Check sheet for the modelled part. Datum: model origin and axes. Units: mm. Give positions to 0.01 mm unless a question says otherwise; leave off trailing zeros. Write each loop counter-clockwise with the first axis right and the second up, starting at its lowest first coordinate (ties: lowest second). Pieces come first, ordered by that corner, then holes. Notation, with made-up numbers: (10.5, 29) -> (18.5, 29) arc R31 cw to (18.5, 56) -> close; hole circle Ø2 at (22, 77). An arc over 180 degrees is marked (long way). Write each question's results on one line, items separated by ' | '. Start each with the question number.
```python
from build123d import *

# Parameters (mm, degrees)
TD_SKETCH_R                             = 0.79248
TL_FEATURE_DEPTH                        = 21.0312
TDF_STD_SKETCH_W                        = 2.09296
TDF_STD_SKETCH_H                        = 2.09296
TDF_STD_FEATURE_DEPTH                   = 22.061040395
ISA_20_STD_FEATURE_DEPTH                = 22.061040395
ISA_20_STD_FEATURE_DEPTH_BACK           = 22.061040395
VW_STD_FEATURE_DEPTH                    = 22.061040395
VW_STD_FEATURE_DEPTH_BACK               = 22.061040395
F_10BA_STD_FEATURE_DEPTH                = 22.061040503
F_10BA_STD_FEATURE_DEPTH_BACK           = 22.061040503
FRO_STD_FEATURE_DEPTH                   = 22.061040395
FRO_STD_FEATURE_DEPTH_BACK              = 22.061040395
C_STD_FEATURE_DEPTH                     = 22.061040395
C_STD_FEATURE_DEPTH_BACK                = 22.061040395
ERW_STD_FEATURE_DEPTH                   = 0.01905
H_STD_FEATURE_REACH                     = 22.896
H_STD_SKETCH_R                          = 0.01905
H_STD_SKETCH_3_R                        = 0.01905
FUNNEL_FINAL_DIAMETRE_STD_FEATURE_DEPTH = 2.499995
FUNNEL_FINAL_DIAMETRE_STD_FEATURE_DRAFT = -22.5
ROUND_BR_STD_FEATURE_START              = -1
ROUND_BR_STD_FEATURE_DEPTH              = 1.009339363


with BuildPart() as part:
    # TD_sketch → TL_feature (new body)
    with BuildSketch(Plane(origin=(0, 0, 0), x_dir=(1, 0, 0), z_dir=(0, 1, 0))):
        with Locations(Location((0, 0, 0), (0, 0, 270))):
            Circle(TD_SKETCH_R)
    extrude(amount=TL_FEATURE_DEPTH)

    # TDF_STD_sketch → TDF_STD_feature (cut, through all)
    with BuildSketch(Plane(origin=(0, 0, 0), x_dir=(1, 0, 0), z_dir=(0, 1, 0))):
        with Locations((-1.4224, 0)):
            Rectangle(TDF_STD_SKETCH_W, TDF_STD_SKETCH_H)
    extrude(amount=TDF_STD_FEATURE_DEPTH, mode=Mode.SUBTRACT)

    # ISA_20_STD_sketch → ISA_20_STD_feature (cut, two sides: drawn at the far end of the back side and taken through both)
    with BuildSketch(Plane(origin=(0, 0, 0), x_dir=(0, 0, -1), z_dir=(1, 0, 0)).offset(-ISA_20_STD_FEATURE_DEPTH_BACK)):
        Polygon((-12.946999885, 73.253224398), (-3.738847997, 21.0312), (-0.03048, 0), (0.03048, 0), (3.738847997, 21.0312), (12.946999885, 73.253224398), (12.946999885, -32.802042202), (-12.946999885, -32.802042202), align=None)
    extrude(amount=ISA_20_STD_FEATURE_DEPTH + ISA_20_STD_FEATURE_DEPTH_BACK, mode=Mode.SUBTRACT)

    # VW_STD_sketch → VW_STD_feature (cut, two sides: drawn at the far end of the back side and taken through both)
    with BuildSketch(Plane(origin=(0, 0, 0), x_dir=(0, 0, -1), z_dir=(1, 0, 0)).offset(-VW_STD_FEATURE_DEPTH_BACK)):
        with BuildLine():
            Line((-70.448918022, 70.704723144), (-20.775394878, 21.0312))
            Line((-20.775394878, 21.0312), (-0.087997439, 0.343802561))
            ThreePointArc((-0.087997439, 0.343802561), (-0.060467299, 0.302600796), (-0.0508, 0.254))
            Line((-0.0508, 0.254), (-0.0508, 0))
            Line((-0.0508, 0), (0.0508, 0))
            Line((0.0508, 0), (0.0508, 0.254))
            ThreePointArc((0.0508, 0.254), (0.060467299, 0.302600796), (0.087997439, 0.343802561))
            Line((0.087997439, 0.343802561), (20.775394878, 21.0312))
            Line((20.775394878, 21.0312), (70.448918022, 70.704723144))
            Line((70.448918022, 70.704723144), (70.448918022, -69.793217099))
            Line((70.448918022, -69.793217099), (-70.448918022, -69.793217099))
            Line((-70.448918022, -69.793217099), (-70.448918022, 70.704723144))
        make_face()
    extrude(amount=VW_STD_FEATURE_DEPTH + VW_STD_FEATURE_DEPTH_BACK, mode=Mode.SUBTRACT)

    # 10BA_STD_sketch → 10BA_STD_feature (cut, two sides: drawn at the far end of the back side and taken through both)
    with BuildSketch(Plane.XY.offset(-F_10BA_STD_FEATURE_DEPTH_BACK)):
        Polygon((-53.216424868, 0), (-0.37592, 0), (-0.29972, 0), (-0.011354365, 0.050846642), (3.688047997, 21.0312), (12.863705374, 73.068938867), (91.245890155, 2.183757568), (25.165759913, -70.885181299), align=None)
    extrude(amount=F_10BA_STD_FEATURE_DEPTH + F_10BA_STD_FEATURE_DEPTH_BACK, mode=Mode.SUBTRACT)

    # FRO_STD_sketch → FRO_STD_feature (cut, two sides: drawn at the far end of the back side and taken through both)
    with BuildSketch(Plane.XY.offset(-FRO_STD_FEATURE_DEPTH_BACK)):
        with BuildLine():
            Line((-0.37592, 52.152138388), (-0.37592, 0.02794))
            ThreePointArc((-0.37592, 0.02794), (-0.367736563, 0.008183437), (-0.34798, 0))
            Line((-0.34798, 0), (51.776218388, 0))
            Line((51.776218388, 0), (-21.9385299, -73.714748288))
            Line((-21.9385299, -73.714748288), (-74.090668288, -21.5626099))
            Line((-74.090668288, -21.5626099), (-0.37592, 52.152138388))
        make_face()
    extrude(amount=FRO_STD_FEATURE_DEPTH + FRO_STD_FEATURE_DEPTH_BACK, mode=Mode.SUBTRACT)

    # C_STD_sketch → C_STD_feature (cut, two sides: drawn at the far end of the back side and taken through both)
    with BuildSketch(Plane(origin=(0, 0, 0), x_dir=(0, 0, -1), z_dir=(1, 0, 0)).offset(-C_STD_FEATURE_DEPTH_BACK)):
        with BuildLine():
            Line((-50.530423385, -12.791040855), (-0.030559272, 0))
            ThreePointArc((-0.030559272, 0), (0, 0.00381), (0.030559272, 0))
            Line((0.030559272, 0), (50.530423385, -12.791040855))
            Line((50.530423385, -12.791040855), (50.530423385, -116.980234183))
            Line((50.530423385, -116.980234183), (-50.530423385, -116.980234183))
            Line((-50.530423385, -116.980234183), (-50.530423385, -12.791040855))
        make_face()
    extrude(amount=C_STD_FEATURE_DEPTH + C_STD_FEATURE_DEPTH_BACK, mode=Mode.SUBTRACT)


with BuildPart() as body_2:
    # ERW_STD_sketch → ERW_STD_feature (new, symmetric)
    with BuildSketch(Plane.XY):
        Polygon((-0.1397, 0.09144), (-0.1397, 0), (-0.32512, 0), (-0.272327091, 0.09144), align=None)
    extrude(amount=ERW_STD_FEATURE_DEPTH, both=True)

    # H_STD_sketch → H_STD_feature (add, up to next)
    with BuildSketch(Plane(origin=(-0.010897713, 0.165804035, 0), x_dir=(0, 0, -1), z_dir=(0.8660254037844415, 0.4999999999999953, 0)), mode=Mode.PRIVATE) as h_std_feature_sk1:
        with Locations(Location((0, 0, 0), (0, 0, 90))):
            Circle(H_STD_SKETCH_R)
    h_std_feature_tool1 = extrude(h_std_feature_sk1.sketch, amount=-H_STD_FEATURE_REACH, mode=Mode.PRIVATE) - body_2.part
    add(h_std_feature_tool1.solids().sort_by_distance((-0.010898, 0.165804, 0))[0])


with BuildPart() as funnel_final_diametre_std_feature_tool:
    # H_STD_sketch<3> → funnel_final_diametre_STD_feature (with draft: the straight prism first)
    with BuildSketch(Plane(origin=(-0.010897713, 0.165804035, 0), x_dir=(0, 0, -1), z_dir=(0.8660254037844415, 0.4999999999999953, 0))):
        with Locations(Location((0, 0, 0), (0, 0, 90))):
            Circle(H_STD_SKETCH_3_R)
    extrude(amount=FUNNEL_FINAL_DIAMETRE_STD_FEATURE_DEPTH)
    # funnel_final_diametre_STD_feature: the draft: its side faces are tilted about the plane it starts from
    funnel_final_diametre_std_feature_sides = [funnel_final_diametre_std_feature_tool.faces().sort_by_distance(p)[0] for p in [
        (1.081156877, 0.774305001, 0),
    ]]
    draft(funnel_final_diametre_std_feature_sides, Plane(origin=(-0.010897713, 0.165804035, 0), x_dir=(0, 0, -1), z_dir=(0.8660254037844415, 0.4999999999999953, 0)), FUNNEL_FINAL_DIAMETRE_STD_FEATURE_DRAFT)


with BuildPart() as body_2_1:
    add(body_2.part)

    # funnel_final_diametre_STD_feature: add funnel_final_diametre_std_feature_tool
    add(funnel_final_diametre_std_feature_tool.part)

    # ROUND_BR_STD_feature: read off the stored shape, not the designer's step
    # ROUND_BR_STD_feature outline → ROUND_BR_STD_feature (cut)
    with BuildSketch(Plane(origin=(0, 0, 0), x_dir=(0.8660254037844362, -0.5000000000000042, 0), z_dir=(0.5000000000000042, 0.8660254037844363, 0)).offset(ROUND_BR_STD_FEATURE_START)):
        with BuildLine():
            Line((-0.281562179, -0.01905), (-0.262512179, -0.01905))
            ThreePointArc((-0.262512179, -0.01905), (-0.275982563, -0.013470384), (-0.281562179, 0))
            Line((-0.281562179, 0), (-0.281562179, -0.01905))
        make_face()
        with BuildLine():
            Line((-0.281562179, 0.01905), (-0.281562179, 0))
            ThreePointArc((-0.281562179, 0), (-0.275982563, 0.013470384), (-0.262512179, 0.01905))
            Line((-0.262512179, 0.01905), (-0.281562179, 0.01905))
        make_face()
    extrude(amount=ROUND_BR_STD_FEATURE_DEPTH, mode=Mode.SUBTRACT)


with BuildPart() as part_1:
    add(part.part)

    # COMBINE_STD_feature: cut body 2
    add(body_2_1.part, mode=Mode.SUBTRACT)


solid = part_1.part
```
Item 1: Section check C-C on y = 2.5. Record the boundary of the cut face in (x, z).
Item 2: Section check A-A on y = 8.5. Record the boundary of the cut face in (x, z).
Item 3: Thickness scan on probe 1 along X at (y, z) = (18.25, 0.05); probe 2 along Z at (x, y) = (0.05, 13.5); probe 3 along Z at (x, y) = (0.1, 3). Record the ranges inside material, lowest first. Write a range as from..to.
Item 4: Section check B-B on x = 0.3. Record the boundary of the cut face in (y, z), then the cut area to 3 significant figures.
Check sheet entries:
1) outline: (-0.38, -0.47) -> (0.42, -0.47) -> (0.42, 0.47) -> (-0.38, 0.47) -> close
2) outline: (-0.38, -0.7) arc R0.79 ccw (long way) to (-0.38, 0.7) -> close
3) probe 1: x = -0.38..0.79 | probe 2: z = -0.79..0.79 | probe 3: z = -0.56..0.56
4) outline: (1.82, -0.35) -> (3.99, -0.73) -> (21.03, -0.73) -> (21.03, 0.73) -> (3.99, 0.73) -> (1.82, 0.35) -> close | area: 27.4 mm^2
